Input: part model. Units: mm. Frame: model coordinates. Round coordinates to 2 decimals unless told otherwise and drop trailing zeros. Loops run counter-clockwise (first coordinate to the right, second up) from the corner with the lowest first, then second, coordinate; pieces in that order, holes last. Notation, with made-up numbers: (-6.75, 2.25) -> (8.25, 2.25) arc R21 ccw to (8.25, 16.25) -> close; hole circle Ø2 at (34.5, 5.25). An arc over 180 degrees is marked (long way). Answer in a Markdown table with one row per item. Add a question column.
Q1. Section A-A, the plane z = 52. Output: boundary loops of the cut face in (x, y).
Q2. Section B-B, the plane x = 2.75. Output: boundary loops of the cut face in (y, z).
Q3. Pin query (flat end, axial travel): pin 1 (1 mm diameter, centred on x = -3, y = 8.5, fed in from +Z); pin 2 (5 mm diameter, centred on x = -2, z = -21, fed in from -Y). Return the tip coordinate at first contact, or that it passes through.
Q4. Ray query, L1, parallel to Z at x = -1.25, y = 12.5; L2, parallel to Y at x = 3.5, z = 6. Return the intervals inside material, ascending. Write a range as from..to.
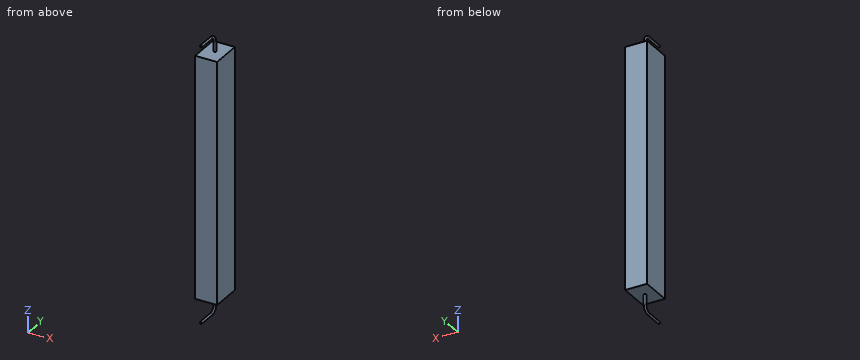
```python
from build123d import *

# Parameters (mm, degrees)
SKETCH_1_W      = 10
SKETCH_1_H      = 14
EXTRUDE_1_DEPTH = 55
SKETCH_3_R      = 0.5


with BuildPart() as part:
    # Эскиз1 → Бобышка-Вытянуть1 (new, symmetric)
    with BuildSketch(Plane.XY):
        with Locations((0, 7)):
            Rectangle(SKETCH_1_W, SKETCH_1_H)
    extrude(amount=EXTRUDE_1_DEPTH, both=True)

    # По траектории1: sweep along a path in Эскиз4
    with BuildLine(Plane(origin=(0, 0, 0), x_dir=(0, 0, -1), z_dir=(1, 0, 0))) as sweep_1_path:
        Line((-62.5, -4), (-62.5, 4))
        ThreePointArc((-62.5, 4), (-61.621320344, 6.121320344), (-59.5, 7))
        Line((-59.5, 7), (-55, 7))
    # Эскиз3 → По траектории1 (sweep)
    with BuildSketch(Plane.XY.offset(55)):
        with Locations((0, 7)):
            Circle(SKETCH_3_R)
    sweep_1 = sweep(path=sweep_1_path.line)

    # Зеркальное отражение1: По траектории1 across plane
    add(sweep_1.mirror(Plane.XY))


solid = part.part
```
Answer block:
| question | item | result |
|---|---|---|
| 1 | outline | (-5, 0) -> (5, 0) -> (5, 14) -> (-5, 14) -> close |
| 2 | outline | (0, -55) -> (14, -55) -> (14, 55) -> (0, 55) -> close |
| 3 | pin 1 | z = 55 |
| 3 | pin 2 | y = 0 |
| 4 | L1 | -55..55 |
| 4 | L2 | 0..14 |
